Geometry: final body of the model. Coordinates: model frame, mm. Face numbers are marked on the shaded views. A direction names the side the tool comes from. Round coordinates to 2 decimals unless told otherwise and drop trailing zeros. Loops run counter-clockwise (first coordinate to the right, second up) from the corner with the lowest first, then second, coordinate; pieces in that order, holes last. Notation, with made-up numbers: (45.5, -15) - (98.5, -15) arc R27 cw to (98.5, 7) - close; hole circle Ø7 at (75, 54). An arc over 180 degrees is marked (long way). Answer as CSV lines item,"result".
from build123d import *

# Parameters (mm, degrees)
SKETCH2_R           = 3.55
BOSS_EXTRUDE1_DEPTH = 3.8
BOSS_EXTRUDE2_DEPTH = 1.4
SKETCH5_R           = 2.549999919
CUT_EXTRUDE1_DEPTH  = 2.5
BOSS_EXTRUDE3_DEPTH = 2.5
SKETCH6_R           = 1.4
CUT_EXTRUDE2_DEPTH  = 12.745554295
SKETCH7_R           = 0.6
CUT_EXTRUDE3_DEPTH  = 12.724676785
CIRPATTERN1_COUNT   = 4
CIRPATTERN2_COUNT   = 4


with BuildPart() as part:
    # Sketch2 → Boss-Extrude1 (new body)
    with BuildSketch(Plane.XY):
        Circle(SKETCH2_R)
    extrude(amount=-BOSS_EXTRUDE1_DEPTH)

    # Sketch4 → Boss-Extrude2 (add)
    with BuildSketch(Plane.XY.offset(-2.4)):
        with BuildLine():
            Line((2.776387215, 2.212277889), (10.622617722, 1.649999976))
            ThreePointArc((10.622617722, 1.649999976), (10.913548722, 0), (10.622617722, -1.649999976))
            Line((10.622617722, -1.649999976), (2.776387215, -2.212277889))
            ThreePointArc((2.776387215, -2.212277889), (3.549999952, 0), (2.776387215, 2.212277889))
        make_face()
    boss_extrude2 = extrude(amount=-BOSS_EXTRUDE2_DEPTH)

    # Sketch5 → Cut-Extrude1 (cut)
    with BuildSketch(Plane.XY):
        Circle(SKETCH5_R)
    extrude(amount=-CUT_EXTRUDE1_DEPTH, mode=Mode.SUBTRACT)

    # Sketch3 → Boss-Extrude3 (add)
    with BuildSketch(Plane.XY):
        with BuildLine():
            Line((-0.244697916, 2.538232164), (0, 2.049999952))
            Line((0, 2.049999952), (0.244697916, 2.538232164))
            ThreePointArc((0.244697916, 2.538232164), (0, 2.549999919), (-0.244697916, 2.538232164))
        make_face()
        with BuildLine():
            Line((0.551635326, 2.489618054), (0.633484824, 1.949665813))
            Line((0.633484824, 1.949665813), (1.017078422, 2.338386424))
            ThreePointArc((1.017078422, 2.338386424), (0.787993311, 2.42519404), (0.551635326, 2.489618054))
        make_face()
        with BuildLine():
            Line((1.29397066, 2.197302783), (1.204959739, 1.6584848))
            Line((1.204959739, 1.6584848), (1.689900206, 1.90964313))
            ThreePointArc((1.689900206, 1.90964313), (1.498852346, 2.06299327), (1.29397066, 2.197302783))
        make_face()
        with BuildLine():
            Line((1.90964313, 1.689900206), (1.6584848, 1.204959739))
            Line((1.6584848, 1.204959739), (2.197302783, 1.29397066))
            ThreePointArc((2.197302783, 1.29397066), (2.06299327, 1.498852346), (1.90964313, 1.689900206))
        make_face()
        with BuildLine():
            Line((2.338386424, 1.017078422), (1.949665813, 0.633484824))
            Line((1.949665813, 0.633484824), (2.489618054, 0.551635326))
            ThreePointArc((2.489618054, 0.551635326), (2.42519404, 0.787993311), (2.338386424, 1.017078422))
        make_face()
        with BuildLine():
            Line((2.538232164, 0.244697916), (2.049999952, 0))
            Line((2.049999952, 0), (2.538232164, -0.244697916))
            ThreePointArc((2.538232164, -0.244697916), (2.549999919, 0), (2.538232164, 0.244697916))
        make_face()
        with BuildLine():
            Line((2.489618054, -0.551635326), (1.949665813, -0.633484824))
            Line((1.949665813, -0.633484824), (2.338386424, -1.017078422))
            ThreePointArc((2.338386424, -1.017078422), (2.42519404, -0.787993311), (2.489618054, -0.551635326))
        make_face()
        with BuildLine():
            Line((2.197302783, -1.29397066), (1.6584848, -1.204959739))
            Line((1.6584848, -1.204959739), (1.90964313, -1.689900206))
            ThreePointArc((1.90964313, -1.689900206), (2.06299327, -1.498852346), (2.197302783, -1.29397066))
        make_face()
        with BuildLine():
            Line((1.689900206, -1.90964313), (1.204959739, -1.6584848))
            Line((1.204959739, -1.6584848), (1.29397066, -2.197302783))
            ThreePointArc((1.29397066, -2.197302783), (1.498852346, -2.06299327), (1.689900206, -1.90964313))
        make_face()
        with BuildLine():
            Line((1.017078422, -2.338386424), (0.633484824, -1.949665813))
            Line((0.633484824, -1.949665813), (0.551635326, -2.489618054))
            ThreePointArc((0.551635326, -2.489618054), (0.787993311, -2.42519404), (1.017078422, -2.338386424))
        make_face()
        with BuildLine():
            Line((0.244697916, -2.538232164), (0, -2.049999952))
            Line((0, -2.049999952), (-0.244697916, -2.538232164))
            ThreePointArc((-0.244697916, -2.538232164), (0, -2.549999919), (0.244697916, -2.538232164))
        make_face()
        with BuildLine():
            Line((-0.551635326, -2.489618054), (-0.633484824, -1.949665813))
            Line((-0.633484824, -1.949665813), (-1.017078422, -2.338386424))
            ThreePointArc((-1.017078422, -2.338386424), (-0.787993311, -2.42519404), (-0.551635326, -2.489618054))
        make_face()
        with BuildLine():
            Line((-1.29397066, -2.197302783), (-1.204959739, -1.6584848))
            Line((-1.204959739, -1.6584848), (-1.689900206, -1.90964313))
            ThreePointArc((-1.689900206, -1.90964313), (-1.498852346, -2.06299327), (-1.29397066, -2.197302783))
        make_face()
        with BuildLine():
            Line((-1.90964313, -1.689900206), (-1.6584848, -1.204959739))
            Line((-1.6584848, -1.204959739), (-2.197302783, -1.29397066))
            ThreePointArc((-2.197302783, -1.29397066), (-2.06299327, -1.498852346), (-1.90964313, -1.689900206))
        make_face()
        with BuildLine():
            Line((-2.338386424, -1.017078422), (-1.949665813, -0.633484824))
            Line((-1.949665813, -0.633484824), (-2.489618054, -0.551635326))
            ThreePointArc((-2.489618054, -0.551635326), (-2.42519404, -0.787993311), (-2.338386424, -1.017078422))
        make_face()
        with BuildLine():
            Line((-2.538232164, -0.244697916), (-2.049999952, 0))
            Line((-2.049999952, 0), (-2.538232164, 0.244697916))
            ThreePointArc((-2.538232164, 0.244697916), (-2.549999919, 0), (-2.538232164, -0.244697916))
        make_face()
        with BuildLine():
            Line((-2.489618054, 0.551635326), (-1.949665813, 0.633484824))
            Line((-1.949665813, 0.633484824), (-2.338386424, 1.017078422))
            ThreePointArc((-2.338386424, 1.017078422), (-2.42519404, 0.787993311), (-2.489618054, 0.551635326))
        make_face()
        with BuildLine():
            Line((-2.197302783, 1.29397066), (-1.6584848, 1.204959739))
            Line((-1.6584848, 1.204959739), (-1.90964313, 1.689900206))
            ThreePointArc((-1.90964313, 1.689900206), (-2.06299327, 1.498852346), (-2.197302783, 1.29397066))
        make_face()
        with BuildLine():
            Line((-1.689900206, 1.90964313), (-1.204959739, 1.6584848))
            Line((-1.204959739, 1.6584848), (-1.29397066, 2.197302783))
            ThreePointArc((-1.29397066, 2.197302783), (-1.498852346, 2.06299327), (-1.689900206, 1.90964313))
        make_face()
        with BuildLine():
            Line((-1.017078422, 2.338386424), (-0.633484824, 1.949665813))
            Line((-0.633484824, 1.949665813), (-0.551635326, 2.489618054))
            ThreePointArc((-0.551635326, 2.489618054), (-0.787993311, 2.42519404), (-1.017078422, 2.338386424))
        make_face()
    extrude(amount=-BOSS_EXTRUDE3_DEPTH)

    # Sketch6 → Cut-Extrude2 (cut, through all)
    with BuildSketch(Plane.XY.offset(-2.5)):
        Circle(SKETCH6_R)
    extrude(amount=-CUT_EXTRUDE2_DEPTH, mode=Mode.SUBTRACT)

    # Sketch7 → Cut-Extrude3 (cut, through all)
    with BuildSketch(Plane.XY.offset(-2.4)):
        with Locations((8.5405208, 0)):
            Circle(SKETCH7_R)
    cut_extrude3 = extrude(amount=-CUT_EXTRUDE3_DEPTH, mode=Mode.SUBTRACT)

    # CirPattern1: Boss-Extrude2 ×4 about axis
    cirpattern1_axis = Axis((0, 0, 0), (0, 0, 1))
    for i in range(1, CIRPATTERN1_COUNT):
        add(boss_extrude2.rotate(cirpattern1_axis, i * 360 / CIRPATTERN1_COUNT))

    # CirPattern2: Cut-Extrude3 ×4 about axis
    cirpattern2_axis = Axis((0, 0, 0), (0, 0, 1))
    for i in range(1, CIRPATTERN2_COUNT):
        add(cut_extrude3.rotate(cirpattern2_axis, i * 360 / CIRPATTERN2_COUNT), mode=Mode.SUBTRACT)


solid = part.part
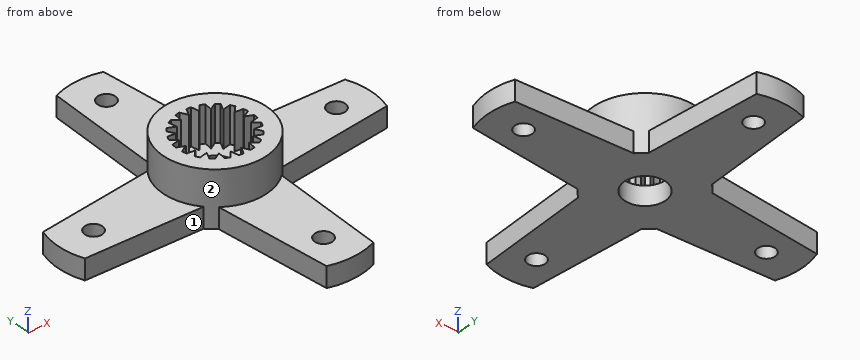
(1) Section B-B (x = -3.25). Output: boundary loops of the cut face in (y, z), and give its area (3 significant figures).
Findings below:
outline,"(-2.18, -3.8) - (2.18, -3.8) - (2.18, -2.4) - (1.43, -2.4) - (1.43, 0) - (-1.43, 0) - (-1.43, -2.4) - (-2.18, -2.4) - close"
area,"13.0 mm2"
(2) Access query for the marked faces 1 and 2. Directions: +Z, -Z, +X, -X, +Y, -Y. A direction counts if a zero-diameter tool reaches every point of the face in a straight line with its end or side. Return the directions, or none.
Findings below:
face 1,"+Z, -Z, -X, -Y"
face 2,"+Z"
(3) Section C-C (y = 4.75). Output: boundary loops of the cut face in (x, z).
Findings below:
outline,"(-2.07, -3.8) - (2.07, -3.8) - (2.07, -2.4) - (-2.07, -2.4) - close"
(4) Section D-D (y = -6). Output: boundary loops of the cut face in (x, z), and give its area (3 significant figures).
Findings below:
outline,"(-1.98, -3.8) - (1.98, -3.8) - (1.98, -2.4) - (-1.98, -2.4) - close"
area,"5.55 mm2"
(5) Pin query (flat end, axial travel): P1, Ø1.4, axis at x = 0, y = -8.54, coming from the -Z side; P2, Ø2, axis at x = -2, z = -1.5, coming from the +Y side; P3, Ø3.5, axis at x = -1, y = -7.5, coming from the +Z side; P4, Ø1, axis at y = -6, z = -2, coming from the +X side. Return the tip coordinate at first contact, or that it passes through.
Findings below:
P1,"z = -3.8"
P2,"y = 10.65"
P3,"z = -2.4"
P4,"x = 2"
(6) Material intervals for line 1 along Z through (x, y) = (-6, 0.75); line 2 along Y through (x, z) = (-0.5, -3.4); line 3 along X through (y, z) = (1, -3.55), sorted ascending.
Findings below:
line 1,"-3.8 to -2.4"
line 2,"-10.89 to -8.87, -8.21 to -1.31, 1.31 to 8.21, 8.87 to 10.89"
line 3,"-10.81 to -0.98, 0.98 to 10.81"
(7) Section A-A (z = -3.5). Output: boundary loops of the cut face in (x, y).
Findings below:
outline,"(-10.62, -1.65) - (-2.78, -2.21) arc R3.55 ccw to (-2.21, -2.78) - (-1.65, -10.62) arc R4.82 ccw to (1.65, -10.62) - (2.21, -2.78) arc R3.55 ccw to (2.78, -2.21) - (10.62, -1.65) arc R4.82 ccw to (10.62, 1.65) - (2.78, 2.21) arc R3.55 ccw to (2.21, 2.78) - (1.65, 10.62) arc R4.82 ccw to (-1.65, 10.62) - (-2.21, 2.78) arc R3.55 ccw to (-2.78, 2.21) - (-10.62, 1.65) arc R4.82 ccw to start; hole circle Ø1.2 at (-8.54, 0); hole circle Ø2.8 at (0, 0); hole circle Ø1.2 at (0, -8.54); hole circle Ø1.2 at (0, 8.54); hole circle Ø1.2 at (8.54, 0)"
